Source: CAD feature listing. Evaluate the final solid. Frame: model axes, mm. Face numbers are marked on the shaded views. A direction names the side the tool comes from. Give positions to 0.01 mm unless a question says otherwise; leave off trailing zeros. Order: outer loops, then holes, each group sorted by start corner. A loop starts at its lowest first (then second) coordinate and runs counter-clockwise, first axis right, second up. Notation, with made-up numbers: M 64,41.25 L 109,41.25 A29 ccw 109,73.25 Z; hole C 43,40 d10. An arc over 180 degrees is marked long. Use CSV: the item, a comma, the result in double quotes. Start each with the question number.
1. Section query C-C, the plane y = 2.75. Return the cut outline in (x, z), plus the area to 3 significant figures.
2. Section query D-D, the plane x = -2. Return the cut outline in (y, z), plus the area to 3 significant figures.
3. Reachability of the marked faces 4 and 5 from +Z, -Z, +X, -X, +Y, -Y: full face, straight path, thin tool, end or side. Return the list, or none.
4. Section query B-B, the plane x = 0. Return the cut outline in (y, z).
5. Pin query (flat end, axial travel): P1, Ø2, axis at x = 2, y = 0.5, coming from the -Z side; P2, Ø1.5, axis at y = 0, z = 2.5, coming from the +X side. Return the tip coordinate at first contact, or that it passes through.
6. Mould query, pull axis X, two halves, no side actions, for the marked faces 1, 2 and 3. Classes: released by +X, released by -X, zero draft, split by the parting line, or undercut.
7. Line query: line 1 along Z through (x, y) = (0, -1); line 2 along Z through (x, y) = (0, 1); line 3 along Y through (x, z) = (-1.6, -1.9). Output: solid intervals per line, ascending. Write a range as [from, to].
8. Section query A-A, the plane z = 0. Return the cut outline in (x, y).
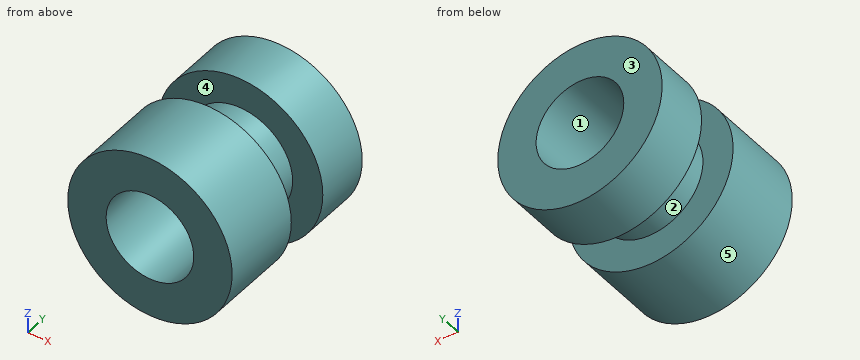
Autodesk Fusion 360 part; units mm, degrees
sketch "Sketch1" plane through (0, 0, 0) normal (0, 0, 1) x (1, 0, 0)
  line L0 (0, 3.3) -> (0, -3.3)
  line L1 (0, 3.3) -> (3, 3.3)
  line L2 (3, 3.3) -> (3, 1.3)
  line L3 (3, 1.3) -> (1.9, 1.3)
  line L4 (1.9, 1.3) -> (1.9, -0.3)
  line L5 (1.9, -0.3) -> (3, -0.3)
  line L6 (3, -0.3) -> (3, -3.3)
  line L7 (0, -3.3) -> (3, -3.3)
  dimension "d2" = 6.6
  dimension "d3" = 3.3
  dimension "d4" = 3
  dimension "d5" = 3
  dimension "d6" = 1.6
  dimension "d7" = 1.9
revolve "Revolve1" add sketch "Sketch1" angle 360 about axis through (0, 3.3, 0) along (0, -1, 0)
sketch "Sketch2" plane through (0, 3.3, 0) normal (0, 1, 0) x (-1, 0, 0)
  circle A0 centre (0, 0) radius 3
  circle A1 centre (0, 0) radius 1.6
  dimension "d9" = 3.2
extrude "Extrude1" cut sketch "Sketch2" against normal through all contours A1
equation "d3 = d2 / 2"
equation "d7 = ( 3.8 / 2 ) * 1 mm"
Result set:
1,outline,"C 0,0 d6; hole C 0,0 d3.2"
1,area,"20.2 mm2"
2,outline,"M -3.3,-2.24 L -0.3,-2.24 L -0.3,2.24 L -3.3,2.24 Z; M 1.3,-2.24 L 3.3,-2.24 L 3.3,2.24 L 1.3,2.24 Z"
2,area,"22.4 mm2"
3,face 4,"none"
3,face 5,"+Y, -Y"
4,outline,"M -3.3,-3 L -0.3,-3 L -0.3,-1.9 L 1.3,-1.9 L 1.3,-3 L 3.3,-3 L 3.3,-1.6 L -3.3,-1.6 Z; M -3.3,1.6 L 3.3,1.6 L 3.3,3 L 1.3,3 L 1.3,1.9 L -0.3,1.9 L -0.3,3 L -3.3,3 Z"
5,P1,"z = -2.65"
5,P2,"x = 2.39"
6,face 1,"undercut"
6,face 2,"split by the parting line"
6,face 3,"zero draft"
7,line 1,"[-3, -1.6], [1.6, 3]"
7,line 2,"[-1.9, -1.6], [1.6, 1.9]"
7,line 3,"[-3.3, -0.3], [1.3, 3.3]"
8,outline,"M -3,-3.3 L -1.6,-3.3 L -1.6,3.3 L -3,3.3 L -3,1.3 L -1.9,1.3 L -1.9,-0.3 L -3,-0.3 Z; M 1.6,-3.3 L 3,-3.3 L 3,-0.3 L 1.9,-0.3 L 1.9,1.3 L 3,1.3 L 3,3.3 L 1.6,3.3 Z"
